```python
from build123d import *

# Parameters (mm, degrees)
EXTRUDE1_DEPTH     = 2.54
EXTRUDE2_DEPTH     = 2
SKETCH4_W          = 45.95
SKETCH4_H          = 18
SKETCH4_W_2        = 41.95
SKETCH4_H_2        = 14
EXTRUDE3_DEPTH     = 5
SKETCH5_W          = 11.95
SKETCH5_H          = 14
EXTRUDE4_DEPTH     = 5
SKETCH6_W          = 2
SKETCH6_H          = 14
CUT_EXTRUDE1_DEPTH = 43.95
CUT_EXTRUDE2_REACH = 9.54
SKETCH7_W          = 8.95
SKETCH7_H          = 14
FILLET1_R          = 2
SKETCH8_W          = 7.54
SKETCH8_H          = 3
EXTRUDE5_DEPTH     = 1
EXTRUDE5_TAPER     = 3
SKETCH9_W          = 7.54
SKETCH9_H          = 3
EXTRUDE6_DEPTH     = 1
EXTRUDE6_TAPER     = 3


with BuildPart() as part:
    # Sketch1 → Extrude1 (new body)
    with BuildSketch(Plane(origin=(0, 0, 0), x_dir=(0, 0, -1), z_dir=(1, 0, 0))):
        Polygon((-62.15, 10), (7.85, 10), (7.85, -10), (-9.2, -10), (-11.2, -8), (-62.15, -8), align=None)
        with BuildLine():
            Line((-6.35, 1.5875), (-6.35, -1.5875))
            ThreePointArc((-6.35, -1.5875), (0, -7.9375), (6.35, -1.5875))
            Line((6.35, -1.5875), (6.35, 1.5875))
            ThreePointArc((6.35, 1.5875), (0, 7.9375), (-6.35, 1.5875))
        make_face(mode=Mode.SUBTRACT)
    extrude(amount=EXTRUDE1_DEPTH)

    # Sketch3 → Extrude2 (add)
    with BuildSketch(Plane.ZY):
        with BuildLine():
            Line((11.2, -8), (11.200000082, 1.5875))
            ThreePointArc((11.200000082, 1.5875), (10.204208676, 6.204222555), (7.393905977, 10))
            Line((7.393905977, 10), (-7.85, 10))
            Line((-7.85, 10), (-7.85, -10))
            Line((-7.85, -10), (9.2, -10))
            Line((9.2, -10), (11.2, -8))
        make_face()
        with BuildLine():
            Line((6.35, 1.5875), (6.35, -1.5875))
            ThreePointArc((6.35, -1.5875), (0, -7.9375), (-6.35, -1.5875))
            Line((-6.35, -1.5875), (-6.35, 1.5875))
            ThreePointArc((-6.35, 1.5875), (0, 7.9375), (6.35, 1.5875))
        make_face(mode=Mode.SUBTRACT)
    extrude(amount=EXTRUDE2_DEPTH)

    # Sketch4 → Extrude3 (add)
    with BuildSketch(Plane.ZY):
        with Locations((39.175, 1)):
            Rectangle(SKETCH4_W, SKETCH4_H)
        with Locations((39.175, 1)):
            Rectangle(SKETCH4_W_2, SKETCH4_H_2, mode=Mode.SUBTRACT)
    extrude(amount=EXTRUDE3_DEPTH)

    # Sketch5 → Extrude4 (add)
    with BuildSketch(Plane.ZY):
        with Locations((39.175, 1)):
            Rectangle(SKETCH5_W, SKETCH5_H)
    extrude(amount=EXTRUDE4_DEPTH)

    # Sketch6 → Cut-Extrude1 (cut)
    with BuildSketch(Plane.XY.offset(62.15)):
        with Locations((-1, 1)):
            Rectangle(SKETCH6_W, SKETCH6_H)
    extrude(amount=-CUT_EXTRUDE1_DEPTH, mode=Mode.SUBTRACT)

    # Sketch7 → Cut-Extrude2 (cut, up to next)
    with BuildSketch(Plane(origin=(2.54, 0, 0), x_dir=(0, 0, -1), z_dir=(1, 0, 0)), mode=Mode.PRIVATE) as cut_extrude2_sk1:
        with Locations((-39.175, 1)):
            Rectangle(SKETCH7_W, SKETCH7_H)
    cut_extrude2_tool1 = extrude(cut_extrude2_sk1.sketch, amount=-CUT_EXTRUDE2_REACH, mode=Mode.PRIVATE) & part.part
    add(cut_extrude2_tool1.solids().sort_by_distance((2.54, 1, 39.175))[0], mode=Mode.SUBTRACT)

    # Fillet1
    fillet1_edges = [part.edges().sort_by_distance(p)[0] for p in [
        (0.27, 10, -7.85),
        (0.27, -10, -7.85),
        (0.27, -10, 9.2),
        (1.27, -8, 11.2),
        (-1, 10, 7.393905977),
        (0, 1, 16.2),
    ]]
    fillet(fillet1_edges, radius=FILLET1_R)

    # Sketch8 → Extrude5 (add)
    with BuildSketch(Plane(origin=(0, 10, 0), x_dir=(1, 0, 0), z_dir=(0, 1, 0))):
        with Locations((-1.23, -22.7)):
            Rectangle(SKETCH8_W, SKETCH8_H)
        with Locations((-1.23, -55.65)):
            Rectangle(SKETCH8_W, SKETCH8_H)
    extrude(amount=EXTRUDE5_DEPTH, taper=EXTRUDE5_TAPER)

    # Sketch9 → Extrude6 (add)
    with BuildSketch(Plane.XZ.offset(8)):
        with Locations((-1.23, 22.7)):
            Rectangle(SKETCH9_W, SKETCH9_H)
    extrude(amount=EXTRUDE6_DEPTH, taper=EXTRUDE6_TAPER)


solid = part.part
```
Verification items for the finished model (mm, model axes). A direction names the side the tool comes from. Round coordinates to 2 decimals unless told otherwise and drop trailing zeros. Order: outer loops, then holes, each group sorted by start corner. A loop starts at its lowest first (then second) coordinate and runs counter-clockwise, first axis right, second up.
1) Cross-section at A-A, the plane z = 0. Record the cut outline in (x, y), plus the area to 3 significant figures.
Geometry says:
outline: (-2, -10) - (2.54, -10) - (2.54, -7.94) - (-2, -7.94) - close; (-2, 7.94) - (2.54, 7.94) - (2.54, 10) - (-2, 10) - close
area: 18.7 mm2
2) Cross-section at D-D, the plane x = -3.5. Give the number of separate pieces and of enclosed holes in the cut face, plus the area to 3 significant figures.
Geometry says:
separate pieces: 1
enclosed holes: 2
area: 416 mm2
3) Cross-section at B-B, the plane y = 3.5. Record the cut outline in (x, z).
Geometry says:
outline: (-5, 16.2) - (-2, 16.2) arc R2 cw to (0, 14.2) - (0, 11.04) - (-2, 11.04) - (-2, 6.06) - (2.54, 6.06) - (2.54, 34.7) - (0, 34.7) - (0, 18.2) - (-5, 18.2) - close; (-5, 33.2) - (-2, 33.2) - (-2, 45.15) - (-5, 45.15) - close; (-5, 60.15) - (-2, 60.15) - (-2, 62.15) - (-5, 62.15) - close; (-2, -7.85) - (2.54, -7.85) - (2.54, -6.06) - (-2, -6.06) - close; (0, 43.65) - (2.54, 43.65) - (2.54, 62.15) - (0, 62.15) - close
4) Depth check by flat-ended pin: pin 1 (2.5 mm diameter, centred on x = -4, y = -2, fed in from -Z); pin 2 (8.5 mm diameter, centred on y = -3.5, z = 11.5, fed in from -X); pin 3 (2.5 mm diameter, centred on x = 0, z = 6, fed in from +Y). Enter the tip coordinate at first touch or a pass-through.
Geometry says:
pin 1: stops at z = 16.2
pin 2: stops at x = -2
pin 3: stops at y = 10
5) Material ranges on line 1 (Z direction, x = -3, y = -3.75); line 2 (Y direction, x = -3, z = 30); line 3 (Z direction, x = 0.5, y = 0), recorded low to high.
Geometry says:
line 1: z = 16.2 to 18.2, 33.2 to 45.15, 60.15 to 62.15
line 2: y = -8 to -6, 8 to 10
line 3: z = -7.85 to -6.35, 6.35 to 34.7, 43.65 to 62.15
6) Tool access check on faces 4 (the flat face through (-3, 1, 33.2)), 5 (the flat face through (0, -8, 18)), 6 (the flat face through (0, 0, -6.35)). Record the directions out of +Z, -Z, +X, -X, +Y, -Y that give a thin tool (end or side, any length) a straight path to the whole face; none if there is none.
Geometry says:
face 4: -X
face 5: +X, -X, -Y
face 6: +X, -X
7) Draft check along Y on faces 1 (the flat face through (-2, 1, 39)), 2 (the cylindrical face through (-1.014, 9.847, 7.365)), 3 (the flat face through (0, 0, -7.85)). Enter one of: +Y half, -Y half, draft (parallel to the pull), parting line (faces both ways), or undercut.
Geometry says:
face 1: undercut
face 2: +Y half
face 3: draft
8) Cross-section at C-C, the plane z = 50.5. Record the cut outline in (x, y), plus the area to 3 significant figures.
Geometry says:
outline: (-5, -8) - (2.54, -8) - (2.54, 10) - (-5, 10) - (-5, 8) - (0, 8) - (0, -6) - (-5, -6) - close
area: 65.7 mm2
